from build123d import *

# Parameters (mm, degrees)
F2_D     = 3.96875
F2_DEPTH = 6.478
F3_SIZE  = 0.79375


with BuildPart() as f1:
    # F0 (on Front) → F1 (revolve)
    with BuildSketch(Plane.XZ):
        with BuildLine():
            Line((0, 6.477), (0, 0))
            Line((0, 0), (41.398825, 0))
            ThreePointArc((41.398825, 0), (43.3832, 1.984375), (45.367575, 0))
            Line((45.367575, 0), (47.752, 0))
            Line((47.752, 0), (47.752, 4.7625))
            Line((47.752, 4.7625), (3.302, 4.7625))
            Line((3.302, 4.7625), (3.302, 6.477))
            Line((3.302, 6.477), (0, 6.477))
        make_face()
        with BuildLine():
            ThreePointArc((45.367575, 0), (43.3832, 1.984375), (41.398825, 0))
            Line((41.398825, 0), (45.367575, 0))
        make_face()
        with BuildLine():
            Line((45.367575, 0), (41.398825, 0))
            ThreePointArc((41.398825, 0), (43.3832, -1.984375), (45.367575, 0))
        make_face()
    revolve(axis=Axis((23.876, 0, 0), (1, 0, 0)))

    # F2 (through all, one way)
    with BuildSketch(Plane(origin=(0, 0, 0), x_dir=(1, 0, 0), z_dir=(0, 1, 0))):
        with Locations((43.3832, 0)):
            Circle(F2_D / 2)
    extrude(amount=-F2_DEPTH, mode=Mode.SUBTRACT)

    # F3
    f3_edges = [f1.edges().sort_by_distance(p)[0] for p in [
        (47.752, 0, -4.7625),
        (0, 0, -6.477),
    ]]
    chamfer(f3_edges, length=F3_SIZE)


solid = f1.part
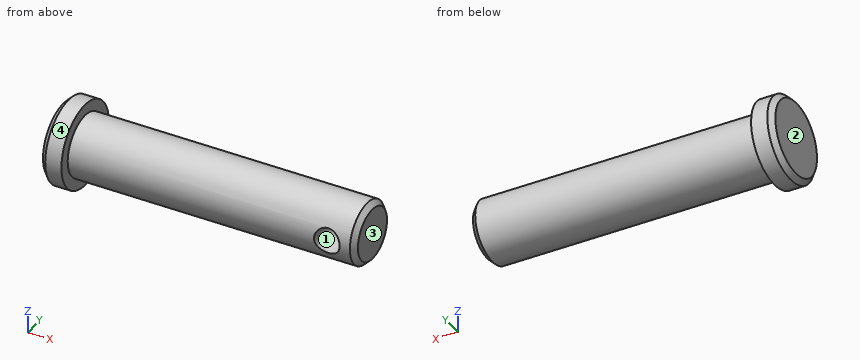
Read the model definition and answer for the solid it produces. Units are mm, in the model's axes. Face numbers are marked on the shaded views. Coordinates: 2 decimals unless noted, no trailing zeros. Loops run counter-clockwise (first coordinate to the right, second up) from the corner with the lowest first, then second, coordinate; pieces in that order, holes last. Notation, with made-up numbers: (52, 31) -> (88, 31) arc R17 ccw to (88, 63) -> close; hole circle Ø3 at (60, 27). An arc over 180 degrees is marked (long way). Answer in a Markdown table with one row per item.
Item 1: For a pull along X with two mould halves and no side action, classify the marked faces 1, 2, 3 and 4 as released by +X, released by -X, zero draft, split by the parting line, or undercut.
Returned:
| item | result |
|---|---|
| face 1 | undercut |
| face 2 | released by -X |
| face 3 | released by +X |
| face 4 | zero draft |
Item 2: Straight lines are drawn through the part: line 1 along X through (y, z) = (-2, 0); line 2 along X through (y, z) = (-5, 2.5); line 3 along Y through (x, z) = (19, 0). For each, find the intervals that lie inside material, in ascending order. Write a range as [from, to].
Returned:
| item | result |
|---|---|
| line 1 | x = [0, 41.4], [45.37, 47.75] |
| line 2 | x = [0, 3.3] |
| line 3 | y = [-4.76, 4.76] |
Item 3: A cutting plane is placed at B-B on x = 21.5. Determine the outline of the cut face in (y, z) (1 decimal), plus the area to 3 significant figures.
Returned:
| item | result |
|---|---|
| outline | circle Ø9.5 at (0, 0) |
| area | 71.3 mm^2 |
Item 4: A cutting plane is placed at A-A on z = 0. Determine the outline of the cut face in (x, y).
Returned:
| item | result |
|---|---|
| outline | (0, -5.68) -> (0.79, -6.48) -> (3.3, -6.48) -> (3.3, -4.76) -> (41.4, -4.76) -> (41.4, 0) arc R1.98 cw to (45.37, 0) -> (45.37, -4.76) -> (46.96, -4.76) -> (47.75, -3.97) -> (47.75, 3.97) -> (46.96, 4.76) -> (3.3, 4.76) -> (3.3, 6.48) -> (0.79, 6.48) -> (0, 5.68) -> close |
Item 5: Each of these flat-tipped pins is pushed along its axis until it touches: P1, Ø5, axis at x = 38, y = 5, coming from the -Z side; P2, Ø6, axis at x = 17, y = 4, coming from the +Z side; P3, Ø2.5, axis at x = 43.38, z = 0, coming from the +Y side. Where does it stop, or does it pass through?
Returned:
| item | result |
|---|---|
| P1 | stops at z = -4.05 |
| P2 | stops at z = 4.66 |
| P3 | stops at y = 4.76 |
